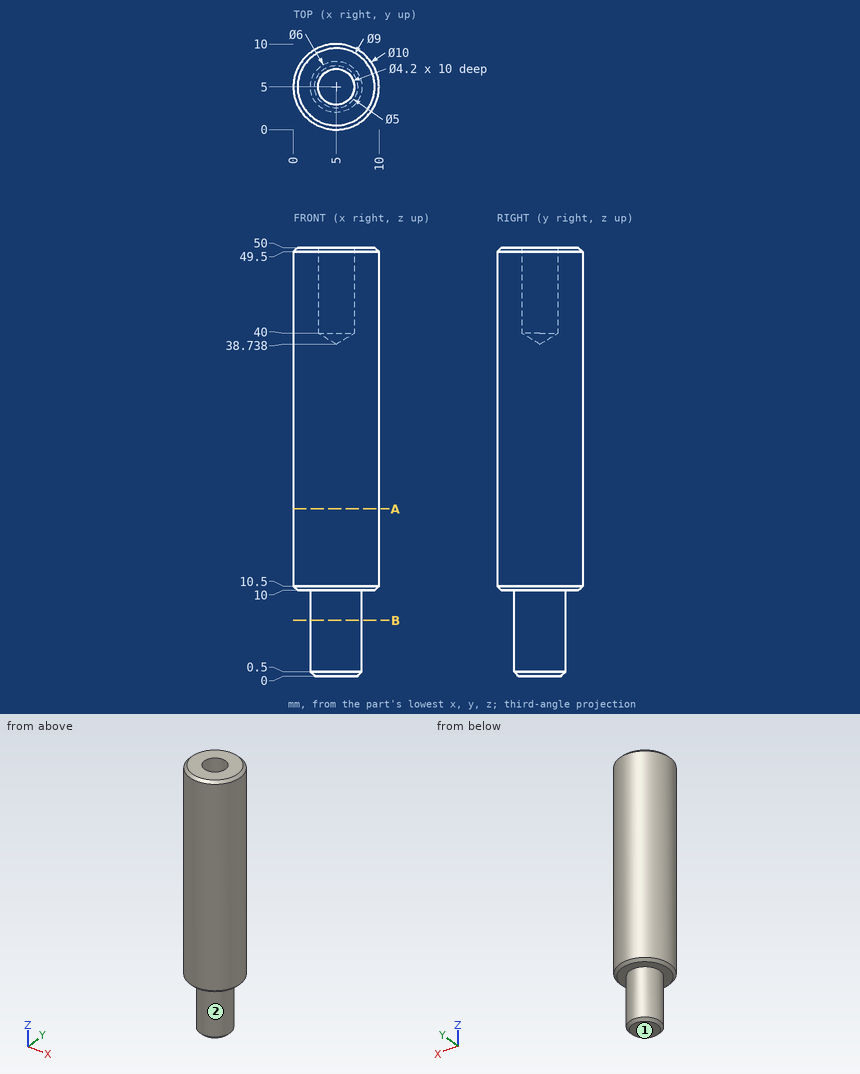
Check sheet for the drawn part. Datum: minimum x, y, z corner. Units: mm. A direction names the side the tool comes from. Coordinates: 2 decimals unless noted, no trailing zeros. Write each loop counter-clockwise with the first axis right and the second up, starting at its lowest first coordinate (ties: lowest second). Pieces come first, ordered by that corner, then holes. Notation, with made-up numbers: M -28.5,53.25 L -6.5,53.25 A33 cw -6.5,81.25 Z; hole C 89.25,32.5 d5. An arc over 180 degrees is marked long. One line per item, written item: value.
Item 1: Access from +Z, -Z, +X, -X, +Y, -Y to the whole of each face (thin tool, end or side, straight path). Record for the marked faces 1 and 2.
Check sheet entries:
face 1: -Z, +X, -X, +Y, -Y
face 2: -Z
Item 2: Scan lines: line 1 along Y through (x, z) = (5, 47.75); line 2 along X through (y, z) = (1, 25.5); line 3 along Z through (x, y) = (8, 7). Record each from-to range of solid material in increasing order.
Check sheet entries:
line 1: y = 0 to 2.9, 7.1 to 10
line 2: x = 2 to 8
line 3: z = 10 to 50
Item 3: Section check A-A, the plane z = 19.5. Record the boundary of the cut face in (x, y).
Check sheet entries:
outline: C 5,5 d10
Item 4: Section check B-B, the plane z = 6.5. Record the boundary of the cut face in (x, y), plus the area to 3 significant figures.
Check sheet entries:
outline: C 5,5 d6
area: 28.3 mm^2
Item 5: Gauge pin test, flat ends, axial feed: pin 1 Ø2 at (x, z) = (8.5, 25) entering from +Y; pin 2 Ø1 at (x, z) = (7.5, 42) entering from -Y. Record the tip position at first contact, or that the pin passes through.
Check sheet entries:
pin 1: stops at y = 9.33
pin 2: stops at y = 0.42
